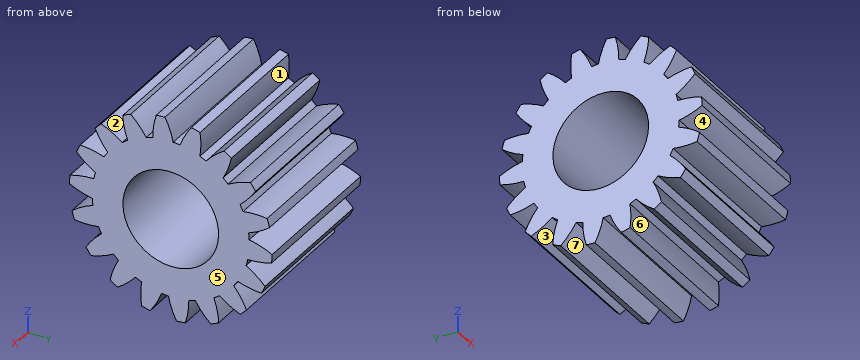
Autodesk Inventor part; units mm, degrees
ref_plane "YZ Plane" through (0, 0, 0) normal (1, 0, 0) x (0, 1, 0)
ref_plane "XZ Plane" through (0, 0, 0) normal (0, 1, 0) x (-1, 0, 0)
ref_plane "XY Plane" through (0, 0, 0) normal (0, 0, 1) x (1, 0, 0)
sketch "Sketch1" plane through (0, 0, 0) normal (1, 0, 0) x (0, 1, 0)
  arc A0 (0.2067, 6.7848) -> (-0.4974, 8.7445) centre (-6.534, 5.4695) ccw
  arc A1 (-0.4974, 8.7445) -> (-1.2576, 8.6679) centre (0, 0) ccw
  arc A2 (-1.2576, 8.6679) -> (-1.5564, 6.6071) centre (5.3112, 6.6633) ccw
  arc A3 (-1.5564, 6.6071) -> (-2.1263, 6.4463) centre (0, 0) ccw
  arc A4 (-2.1263, 6.4463) -> (-3.4581, 8.047) centre (-8.0107, 2.9049) ccw
  arc A5 (-3.4581, 8.047) -> (-4.1463, 7.715) centre (0, 0) ccw
  arc A6 (-4.1463, 7.715) -> (-3.7223, 5.6763) centre (2.7119, 8.078) ccw
  arc A7 (-3.7223, 5.6763) -> (-4.2029, 5.3303) centre (0, 0) ccw
  arc A8 (-4.2029, 5.3303) -> (-6.0018, 6.379) centre (-8.5211, -0.0101) ccw
  arc A9 (-6.0018, 6.379) -> (-6.535, 5.8316) centre (0, 0) ccw
  arc A10 (-6.535, 5.8316) -> (-5.4392, 4.0609) centre (-0.2145, 8.5184) ccw
  arc A11 (-5.4392, 4.0609) -> (-5.7725, 3.5714) centre (0, 0) ccw
  arc A12 (-5.7725, 3.5714) -> (-7.8216, 3.9415) centre (-8.0037, -2.9239) ccw
  arc A13 (-7.8216, 3.9415) -> (-8.1354, 3.2448) centre (0, 0) ccw
  arc A14 (-8.1354, 3.2448) -> (-6.5001, 1.9557) centre (-3.115, 7.9313) ccw
  arc A15 (-6.5001, 1.9557) -> (-6.6458, 1.3817) centre (0, 0) ccw
  arc A16 (-6.6458, 1.3817) -> (-8.698, 1.0287) centre (-6.521, -5.485) ccw
  arc A17 (-8.698, 1.0287) -> (-8.7546, 0.2667) centre (0, 0) ccw
  arc A18 (-8.7546, 0.2667) -> (-6.777, -0.3854) centre (-5.6398, 6.3876) ccw
  arc A19 (-6.777, -0.3854) -> (-6.7176, -0.9746) centre (0, 0) ccw
  arc A20 (-6.7176, -0.9746) -> (-8.5253, -2.0083) centre (-4.2518, -7.3845) ccw
  arc A21 (-8.5253, -2.0083) -> (-8.3178, -2.7436) centre (0, 0) ccw
  arc A22 (-8.3178, -2.7436) -> (-6.2364, -2.6801) centre (-7.4844, 4.0734) ccw
  arc A23 (-6.2364, -2.6801) -> (-5.9791, -3.2134) centre (0, 0) ccw
  arc A24 (-5.9791, -3.2134) -> (-7.3243, -4.803) centre (-1.4697, -8.3934) ccw
  arc A25 (-7.3243, -4.803) -> (-6.8778, -5.423) centre (0, 0) ccw
  arc A26 (-6.8778, -5.423) -> (-4.9437, -4.6514) centre (-8.4262, 1.268) ccw
  arc A27 (-4.9437, -4.6514) -> (-4.5195, -5.0646) centre (0, 0) ccw
  arc A28 (-4.5195, -5.0646) -> (-5.2399, -7.0184) centre (1.4896, -8.3899) ccw
  arc A29 (-5.2399, -7.0184) -> (-4.6082, -7.4483) centre (0, 0) ccw
  arc A30 (-4.6082, -7.4483) -> (-3.0547, -6.0618) centre (-8.3517, -1.6904) ccw
  arc A31 (-3.0547, -6.0618) -> (-2.5147, -6.3049) centre (0, 0) ccw
  arc A32 (-2.5147, -6.3049) -> (-2.5234, -8.3872) centre (4.2693, -7.3744) ccw
  arc A33 (-2.5234, -8.3872) -> (-1.7828, -8.5753) centre (0, 0) ccw
  arc A34 (-1.7828, -8.5753) -> (-0.7972, -6.741) centre (-7.2699, -4.445) ccw
  arc A35 (-0.7972, -6.741) -> (-0.2067, -6.7848) centre (0, 0) ccw
  arc A36 (-0.2067, -6.7848) -> (0.4974, -8.7445) centre (6.534, -5.4695) ccw
  arc A37 (0.4974, -8.7445) -> (1.2576, -8.6679) centre (0, 0) ccw
  arc A38 (1.2576, -8.6679) -> (1.5564, -6.6071) centre (-5.3112, -6.6633) ccw
  arc A39 (1.5564, -6.6071) -> (2.1263, -6.4463) centre (0, 0) ccw
  arc A40 (2.1263, -6.4463) -> (3.4581, -8.047) centre (8.0107, -2.9049) ccw
  arc A41 (3.4581, -8.047) -> (4.1463, -7.715) centre (0, 0) ccw
  arc A42 (4.1463, -7.715) -> (3.7223, -5.6763) centre (-2.7119, -8.078) ccw
  arc A43 (3.7223, -5.6763) -> (4.2029, -5.3303) centre (0, 0) ccw
  arc A44 (4.2029, -5.3303) -> (6.0018, -6.379) centre (8.5211, 0.0101) ccw
  arc A45 (6.0018, -6.379) -> (6.535, -5.8316) centre (0, 0) ccw
  arc A46 (6.535, -5.8316) -> (5.4392, -4.0609) centre (0.2145, -8.5184) ccw
  arc A47 (5.4392, -4.0609) -> (5.7725, -3.5714) centre (0, 0) ccw
  arc A48 (5.7725, -3.5714) -> (7.8216, -3.9415) centre (8.0037, 2.9239) ccw
  arc A49 (7.8216, -3.9415) -> (8.1354, -3.2448) centre (0, 0) ccw
  arc A50 (8.1354, -3.2448) -> (6.5001, -1.9557) centre (3.115, -7.9313) ccw
  arc A51 (6.5001, -1.9557) -> (6.6458, -1.3817) centre (0, 0) ccw
  arc A52 (6.6458, -1.3817) -> (8.698, -1.0287) centre (6.521, 5.485) ccw
  arc A53 (8.698, -1.0287) -> (8.7546, -0.2667) centre (0, 0) ccw
  arc A54 (8.7546, -0.2667) -> (6.777, 0.3854) centre (5.6398, -6.3876) ccw
  arc A55 (6.777, 0.3854) -> (6.7176, 0.9746) centre (0, 0) ccw
  arc A56 (6.7176, 0.9746) -> (8.5253, 2.0083) centre (4.2518, 7.3845) ccw
  arc A57 (8.5253, 2.0083) -> (8.3178, 2.7436) centre (0, 0) ccw
  arc A58 (8.3178, 2.7436) -> (6.2364, 2.6801) centre (7.4844, -4.0734) ccw
  arc A59 (6.2364, 2.6801) -> (5.9791, 3.2134) centre (0, 0) ccw
  arc A60 (5.9791, 3.2134) -> (7.3243, 4.803) centre (1.4697, 8.3934) ccw
  arc A61 (7.3243, 4.803) -> (6.8778, 5.423) centre (0, 0) ccw
  arc A62 (6.8778, 5.423) -> (4.9437, 4.6514) centre (8.4262, -1.268) ccw
  arc A63 (4.9437, 4.6514) -> (4.5195, 5.0646) centre (0, 0) ccw
  arc A64 (4.5195, 5.0646) -> (5.2399, 7.0184) centre (-1.4896, 8.3899) ccw
  arc A65 (5.2399, 7.0184) -> (4.6082, 7.4483) centre (0, 0) ccw
  arc A66 (4.6082, 7.4483) -> (3.0547, 6.0618) centre (8.3517, 1.6904) ccw
  arc A67 (3.0547, 6.0618) -> (2.5147, 6.3049) centre (0, 0) ccw
  arc A68 (2.5147, 6.3049) -> (2.5234, 8.3872) centre (-4.2693, 7.3744) ccw
  arc A69 (2.5234, 8.3872) -> (1.7828, 8.5753) centre (0, 0) ccw
  arc A70 (1.7828, 8.5753) -> (0.7972, 6.741) centre (7.2699, 4.445) ccw
  arc A71 (0.7972, 6.741) -> (0.2067, 6.7848) centre (0, 0) ccw
  point P0 (0, 0)
extrude "Extrusion1" add sketch "Sketch1" along normal blind 12.7
sketch "Sketch2" plane through (12.7, 0, 0) normal (1, 0, 0) x (0, 0, -1)
  arc A0 (-6.741, 0.7972) -> (-6.7848, 0.2067) centre (0, 0) ccw
  circle A1 centre (0, 0) radius 4.1275
  dimension "d2" = 8.255
extrude "Extrusion2" cut sketch "Sketch2" against normal through all
properties part number "Gear"
Geometry check sheet. Reference: the model listing, model coordinates, mm. Face numbers are marked on the shaded views. A direction names the side the tool comes from. Coordinates: 2 decimals unless noted, no trailing zeros. Write each loop counter-clockwise with the first axis right and the second up, starting at its lowest first coordinate (ties: lowest second). Pieces come first, ordered by that corner, then holes. Notation, with made-up numbers: M 33.25,15 L 45.25,15 A26 cw 45.25,29 Z; hole C 32,38.5 d7. An arc over 180 degrees is marked long. Answer as a JSON object with one key per item and string values.
1. Go/stop test with flat-tipped pins: pin 1 Ø6 at (x, y) = (8.5, -4.5) entering from -Z; pin 2 Ø3 at (y, z) = (1, -1.5) entering from -X; pin 3 Ø1 at (x, y) = (2, 1) entering from -Z. Record where each tip stops, or that it passes through.
Answers below:
{"pin 1": "stops at z = -8.58", "pin 2": "passes through", "pin 3": "stops at z = -8.74"}
2. Draft check along Y on the marked faces 4, 5, 6 and 7. Enter one of: released by +Y, released by -Y, zero draft, split by the parting line, or undercut.
Answers below:
{"face 4": "released by -Y", "face 5": "zero draft", "face 6": "undercut", "face 7": "undercut"}
3. Section check A-A, the plane z = 0. Enter the section's corners in (x, y), plus the area to 3 significant figures.
Answers below:
{"outline": "M 0,-8.16 L 12.7,-8.16 L 12.7,-4.13 L 0,-4.13 Z; M 0,4.13 L 12.7,4.13 L 12.7,8.16 L 0,8.16 Z", "area": "102 mm²"}
4. Scan lines: L1, parallel to Z at x = 0.75, y = 8; L2, parallel to Y at x = 10.75, z = -7.5; L3, parallel to Z at x = 6.25, y = -4.75. Record each from-to range of solid material in increasing order.
Answers below:
{"L1": "z = -3.57 to -3.1, -1.22 to 0.06, 1.63 to 2.77", "L2": "y = -2.6 to -1.12, -0.03 to 1.51, 2.91 to 4.13", "L3": "z = -7.36 to -5.52, -4.85 to 5.73"}
5. Tool access check on the marked faces 1, 2 and 3. Record the directions out of +Z, -Z, +X, -X, +Y, -Y that give a thin tool (end or side, any length) a straight path to the whole face; none if there is none.
Answers below:
{"face 1": "+X, -X", "face 2": "+Z, +X, -X", "face 3": "-Z, +X, -X"}
